Could you check a few things on this model? Use its own coordinates, in mm. A direction names the side the tool comes from. Coordinates: 2 decimals unless noted, no trailing zeros. Write each loop counter-clockwise with the first axis right and the second up, starting at its lowest first coordinate (ties: lowest second). Pieces come first, ordered by that corner, then holes. Notation, with made-up numbers: (43.5, 20.5) - (94.5, 20.5) arc R31 ccw to (94.5, 51.5) - close; hole circle Ø11 at (27, 71.5). An arc over 180 degrees is marked (long way). Answer as a JSON object with one key per item and string values. Group by question number.
1) On a 3-axis mill with a long thin cutter (end or side, diameter ignored), from which of +Z, -Z, +X, -X, +Y, -Y can I reach the whole of each face in a straight line? I mean faces 5 (the flat face through (-23, 5, 3)), 6 (the flat face through (10, 17, 2)), 7 (the flat face through (0, 12.5, 4)), 8 (the flat face through (23, -5, 3)), 9 (the flat face through (-23, -5, 3)). Say none if no direction works.
2) If we section it at B-B (y = 0): Write out the boundary of the cut face in (x, z), plus the area to 3 significant figures.
3) If we section it at A-A (x = 0): Write out the boundary of the cut face in (y, z), plus the area to 4 significant figures.
4) If we section it at C-C (y = -10): Write out the boundary of the cut face in (x, z).
5) If we section it at D-D (x = 23.5): Write out the boundary of the cut face in (y, z), plus the area to 3 significant figures.
6) Please list where these lines run through material, in increasing order: line 1 along Y through (x, z) = (-1, 5.75); line 2 along X through (y, z) = (9.5, 5.75); line 3 along X through (y, z) = (6.5, 2.25).
7) We'd pull the mould along Y, two halves only. Please class faces 1 (the flat face through (23, 5, 3)), 2 (the flat face through (0, -13, 0)), 3 (the cylindrical face through (14.036, -14.247, 3.451)), 4 (the cylindrical face through (10, -9, 1)): released by +Y, released by -Y, zero draft, split by the parting line, or undercut.
8) Will these pins go through, and if not, where does the flat tip stop? pin 1 Ø0.9 at (x, y) = (-12.5, 17.5) entering from +Z; pin 2 Ø2 at (x, z) = (21.5, 3.5) entering from +Y; pin 3 Ø4 at (y, z) = (15, 2.5) entering from +X; pin 4 Ø1 at (x, y) = (-10, 1) entering from +Z.
```python
from build123d import *

# Parameters (mm, degrees)
SKETCH2_R           = 20
SKETCH2_W           = 25
SKETCH2_H           = 25
SKETCH2_R_2         = 11.8
SKETCH2_R_3         = 1
BOSS_EXTRUDE1_DEPTH = 2
SKETCH2_3_R         = 20
SKETCH2_3_W         = 25
SKETCH2_3_H         = 25
BOSS_EXTRUDE2_DEPTH = 7
SKETCH4_R           = 1.2
BOSS_EXTRUDE3_DEPTH = 7
CUT_EXTRUDE8_START  = -7
SKETCH5_R           = 1.2
CUT_EXTRUDE8_DEPTH  = 7
SKETCH8_W           = 30
SKETCH8_H           = 7
BOSS_EXTRUDE5_DEPTH = 2.5
SKETCH9_W           = 30
SKETCH9_H           = 1.472120536
CUT_EXTRUDE9_DEPTH  = 12.5
BOSS_EXTRUDE6_DEPTH = 3


with BuildPart() as part:
    # Sketch2 → Boss-Extrude1 (new body)
    # profile 1 of 2: a face of its own
    with BuildSketch(Plane(origin=(0, 0, 0), x_dir=(0, 1, 0), z_dir=(0, 0, 1))):
        with Locations(Location((0, 0, 0), (0, 0, 270))):
            Circle(SKETCH2_R)
        Rectangle(SKETCH2_W, SKETCH2_H, mode=Mode.SUBTRACT)
    # profile 2 of 2: a face of its own
    with BuildSketch(Plane(origin=(0, 0, 0), x_dir=(0, 1, 0), z_dir=(0, 0, 1))):
        Rectangle(SKETCH2_W, SKETCH2_H)
        with Locations(Location((0, 0, 0), (0, 0, 270))):
            Circle(SKETCH2_R_2, mode=Mode.SUBTRACT)
        with Locations(Location((-10, -10, 0), (0, 0, 270))):
            Circle(SKETCH2_R_3, mode=Mode.SUBTRACT)
        with Locations(Location((10, -10, 0), (0, 0, 270))):
            Circle(SKETCH2_R_3, mode=Mode.SUBTRACT)
        with Locations(Location((10, 10, 0), (0, 0, 270))):
            Circle(SKETCH2_R_3, mode=Mode.SUBTRACT)
        with Locations(Location((-10, 10, 0), (0, 0, 270))):
            Circle(SKETCH2_R_3, mode=Mode.SUBTRACT)
    extrude(amount=BOSS_EXTRUDE1_DEPTH)

    # Sketch2<3> → Boss-Extrude2 (add)
    with BuildSketch(Plane(origin=(0, 0, 0), x_dir=(0, 1, 0), z_dir=(0, 0, 1))):
        with Locations(Location((0, 0, 0), (0, 0, 270))):
            Circle(SKETCH2_3_R)
        Rectangle(SKETCH2_3_W, SKETCH2_3_H, mode=Mode.SUBTRACT)
    extrude(amount=BOSS_EXTRUDE2_DEPTH)

    # Sketch4 → Boss-Extrude3 (add)
    # profile 1 of 4: a face of its own
    with BuildSketch(Plane(origin=(0, 0, 0), x_dir=(1, 0, 0), z_dir=(0, 0, -1))):
        with BuildLine():
            ThreePointArc((19.364916731, 5), (20, 0), (19.364916731, -5))
            Line((19.364916731, -5), (27, -5))
            ThreePointArc((27, -5), (32, 0), (27, 5))
            Line((27, 5), (19.364916731, 5))
        make_face()
        with Locations(Location((27, 0, 0), (0, 0, 180))):
            Circle(SKETCH4_R, mode=Mode.SUBTRACT)
    # profile 2 of 4: a face of its own
    with BuildSketch(Plane(origin=(0, 0, 0), x_dir=(1, 0, 0), z_dir=(0, 0, -1))):
        with BuildLine():
            ThreePointArc((-5, 19.364916731), (0, 20), (5, 19.364916731))
            Line((5, 19.364916731), (5, 27))
            ThreePointArc((5, 27), (0, 32), (-5, 27))
            Line((-5, 27), (-5, 19.364916731))
        make_face()
        with Locations(Location((0, 27, 0), (0, 0, 180))):
            Circle(SKETCH4_R, mode=Mode.SUBTRACT)
    # profile 3 of 4: a face of its own
    with BuildSketch(Plane(origin=(0, 0, 0), x_dir=(1, 0, 0), z_dir=(0, 0, -1))):
        with BuildLine():
            Line((5, -27), (5, -19.364916731))
            ThreePointArc((5, -19.364916731), (0, -20), (-5, -19.364916731))
            Line((-5, -19.364916731), (-5, -27))
            ThreePointArc((-5, -27), (0, -32), (5, -27))
        make_face()
        with Locations(Location((0, -27, 0), (0, 0, 180))):
            Circle(SKETCH4_R, mode=Mode.SUBTRACT)
    # profile 4 of 4: a face of its own
    with BuildSketch(Plane(origin=(0, 0, 0), x_dir=(1, 0, 0), z_dir=(0, 0, -1))):
        with BuildLine():
            ThreePointArc((-19.364916731, -5), (-20, 0), (-19.364916731, 5))
            Line((-19.364916731, 5), (-27, 5))
            ThreePointArc((-27, 5), (-32, 0), (-27, -5))
            Line((-27, -5), (-19.364916731, -5))
        make_face()
        with Locations(Location((-27, 0, 0), (0, 0, 180))):
            Circle(SKETCH4_R, mode=Mode.SUBTRACT)
    extrude(amount=-BOSS_EXTRUDE3_DEPTH)

    # Sketch5 → Cut-Extrude8 (cut)
    with BuildSketch(Plane.XY.offset(7).offset(CUT_EXTRUDE8_START)):
        with BuildLine():
            Line((-12.5, 15.612494996), (-12.5, 15.5))
            Line((-12.5, 15.5), (12.5, 15.5))
            Line((12.5, 15.5), (12.5, 15.612494996))
            ThreePointArc((12.5, 15.612494996), (8.948891955, 17.886233052), (5, 19.364916731))
            Line((5, 19.364916731), (5, 27))
            ThreePointArc((5, 27), (0, 32), (-5, 27))
            Line((-5, 27), (-5, 19.364916731))
            ThreePointArc((-5, 19.364916731), (-8.948891955, 17.886233052), (-12.5, 15.612494996))
        make_face()
        with Locations((0, 27)):
            Circle(SKETCH5_R, mode=Mode.SUBTRACT)
    extrude(amount=CUT_EXTRUDE8_DEPTH, mode=Mode.SUBTRACT)

    # Sketch8 → Boss-Extrude5 (add)
    with BuildSketch(Plane(origin=(0, 15.5, 0), x_dir=(-1, 0, 0), z_dir=(0, 1, 0))):
        with Locations((0, 3.5)):
            Rectangle(SKETCH8_W, SKETCH8_H)
    extrude(amount=-BOSS_EXTRUDE5_DEPTH)

    # Sketch9 → Cut-Extrude9 (cut)
    with BuildSketch(Plane.XY.offset(7)):
        with Locations((0, 16.236060268)):
            Rectangle(SKETCH9_W, SKETCH9_H)
    extrude(amount=-CUT_EXTRUDE9_DEPTH, mode=Mode.SUBTRACT)

    # Sketch8<5> → Boss-Extrude6 (add)
    with BuildSketch(Plane(origin=(0, 15.5, 0), x_dir=(-1, 0, 0), z_dir=(0, 1, 0))):
        with BuildLine():
            Line((-10, 3.5), (-11.5, 3.5))
            Line((-11.5, 3.5), (-11.651471863, 3.348528137))
            ThreePointArc((-11.651471863, 3.348528137), (-11.391344561, 2.959220119), (-11.3, 2.5))
            ThreePointArc((-11.3, 2.5), (-11.651471863, 1.651471863), (-12.5, 1.3))
            Line((-12.5, 1.3), (-12.5, 0))
            Line((-12.5, 0), (-10, 0))
            Line((-10, 0), (-10, 3.5))
        make_face()
        with BuildLine():
            ThreePointArc((-12.5, 1.3), (-12.959220119, 1.391344561), (-13.348528137, 1.651471863))
            Line((-13.348528137, 1.651471863), (-15, 0))
            Line((-15, 0), (-12.5, 0))
            Line((-12.5, 0), (-12.5, 1.3))
        make_face()
        with BuildLine():
            ThreePointArc((-13.348528137, 1.651471863), (-13.608655439, 2.959220119), (-12.5, 3.7))
            Line((-12.5, 3.7), (-12.5, 5))
            Line((-12.5, 5), (-15, 5))
            Line((-15, 5), (-15, 0))
            Line((-15, 0), (-13.348528137, 1.651471863))
        make_face()
        with BuildLine():
            ThreePointArc((-12.5, 3.7), (-12.153589838, 3.648912529), (-11.836675042, 3.5))
            Line((-11.836675042, 3.5), (-11.5, 3.5))
            Line((-11.5, 3.5), (-10, 5))
            Line((-10, 5), (-12.5, 5))
            Line((-12.5, 5), (-12.5, 3.7))
        make_face()
        Polygon((-10, 5), (-11.5, 3.5), (-10, 3.5), align=None)
        with BuildLine():
            Line((11.836675042, 3.5), (10, 3.5))
            Line((10, 3.5), (10, 0))
            Line((10, 0), (12.5, 0))
            Line((12.5, 0), (12.5, 1.3))
            ThreePointArc((12.5, 1.3), (11.351087471, 2.153589838), (11.836675042, 3.5))
        make_face()
        with BuildLine():
            Line((10, 5), (10, 3.5))
            Line((10, 3.5), (11.836675042, 3.5))
            ThreePointArc((11.836675042, 3.5), (12.153589838, 3.648912529), (12.5, 3.7))
            Line((12.5, 3.7), (12.5, 5))
            Line((12.5, 5), (10, 5))
        make_face()
        with BuildLine():
            Line((15, 5), (12.5, 5))
            Line((12.5, 5), (12.5, 3.7))
            ThreePointArc((12.5, 3.7), (13.348528137, 3.348528137), (13.7, 2.5))
            ThreePointArc((13.7, 2.5), (13.348528137, 1.651471863), (12.5, 1.3))
            Line((12.5, 1.3), (12.5, 0))
            Line((12.5, 0), (15, 0))
            Line((15, 0), (15, 5))
        make_face()
    extrude(amount=BOSS_EXTRUDE6_DEPTH)


solid = part.part
```
Here are the results:
{
 "1": {"face 5": "+Z, -Z, -X, +Y", "face 6": "+Z, -Z, +Y", "face 7": "+Z", "face 8": "+Z, -Z, +X, -Y", "face 9": "+Z, -Z, -X, -Y"},
 "2": {"outline": "(-32, 0) - (-28.2, 0) - (-28.2, 7) - (-32, 7) - close; (-25.8, 0) - (-11.8, 0) - (-11.8, 2) - (-12.5, 2) - (-12.5, 7) - (-25.8, 7) - close; (11.8, 0) - (25.8, 0) - (25.8, 7) - (12.5, 7) - (12.5, 2) - (11.8, 2) - close; (28.2, 0) - (32, 0) - (32, 7) - (28.2, 7) - close", "area": "242 mm²"},
 "3": {"outline": "(-32, 0) - (-28.2, 0) - (-28.2, 7) - (-32, 7) - close; (-25.8, 0) - (-11.8, 0) - (-11.8, 2) - (-12.5, 2) - (-12.5, 7) - (-25.8, 7) - close; (11.8, 0) - (15.5, 0) - (15.5, 7) - (12.5, 7) - (12.5, 2) - (11.8, 2) - close", "area": "143.5 mm²"},
 "4": {"outline": "(-17.32, 0) - (-11, 0) - (-11, 2) - (-12.5, 2) - (-12.5, 7) - (-17.32, 7) - close; (-9, 0) - (-6.26, 0) - (-6.26, 2) - (-9, 2) - close; (6.26, 0) - (9, 0) - (9, 2) - (6.26, 2) - close; (11, 0) - (17.32, 0) - (17.32, 7) - (12.5, 7) - (12.5, 2) - (11, 2) - close"},
 "5": {"outline": "(-5, 0) - (5, 0) - (5, 7) - (-5, 7) - close", "area": "70.0 mm²"},
 "6": {"line 1": "y = -31.9 to -27.66, -26.34 to -12.5, 12.5 to 15.5", "line 2": "x = -17.6 to -12.5, 12.5 to 17.6", "line 3": "x = -18.91 to -12.5, 12.5 to 18.91"},
 "7": {"face 1": "released by +Y", "face 2": "zero draft", "face 3": "released by -Y", "face 4": "undercut"},
 "8": {"pin 1": "stops at z = 5", "pin 2": "stops at y = 5", "pin 3": "stops at x = 15.2", "pin 4": "passes through"}
}
